Work out the finished part from the listing and answer in its coordinate system (mm). Give positions to 0.01 mm unless a question says otherwise; leave off trailing zeros. Loops run counter-clockwise (first coordinate to the right, second up) from the corner with the lowest first, then second, coordinate; pieces in that order, holes last. Notation, with made-up numbers: (34, 24.25) - (91, 24.25) arc R28 ccw to (91, 54.25) - close; hole circle Ø9 at (-15.75, 81). An arc over 180 degrees is marked (long way). One line per question, with ' | ' between items.
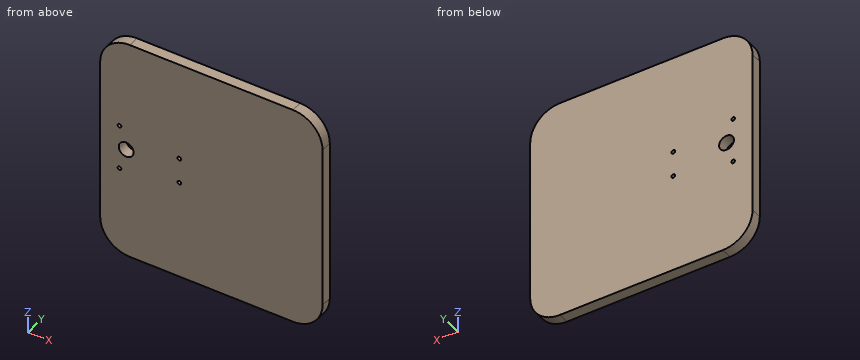
from build123d import *

# Parameters (mm, degrees)
SKETCH1_W               = 150
SKETCH1_H               = 150
BOSS_EXTRUDE1_DEPTH     = 7.5
CUT_EXTRUDE1_DEPTH      = 107.330851591
CUT_EXTRUDE1_DEPTH_BACK = 107.330851591
SKETCH2_R               = 1.25
SKETCH2_R_2             = 5
FILLET1_R               = 20


with BuildPart() as part:
    # Sketch1 → Boss-Extrude1 (new body)
    with BuildSketch(Plane(origin=(0, 0, 0), x_dir=(1, 0, 0), z_dir=(0, 1, 0))):
        Rectangle(SKETCH1_W, SKETCH1_H)
    extrude(amount=BOSS_EXTRUDE1_DEPTH)

    # Sketch2 → Cut-Extrude1 (cut, two sides: drawn at the far end of the back side and taken through both)
    with BuildSketch(Plane(origin=(0, 7.5, 0), x_dir=(1, 0, 0), z_dir=(0, 1, 0)).offset(-CUT_EXTRUDE1_DEPTH_BACK)):
        with Locations(Location((-61.985746634, -15.05, 0), (0, 0, 270))):
            Circle(SKETCH2_R)
        with Locations(Location((-61.985746634, 15.05, 0), (0, 0, 270))):
            Circle(SKETCH2_R)
        with Locations(Location((-21.585746634, 8.55, 0), (0, 0, 270))):
            Circle(SKETCH2_R)
        with Locations(Location((-21.585746634, -8.55, 0), (0, 0, 270))):
            Circle(SKETCH2_R)
        with Locations(Location((-57.485746634, 0, 0), (0, 0, 270))):
            Circle(SKETCH2_R_2)
    extrude(amount=CUT_EXTRUDE1_DEPTH + CUT_EXTRUDE1_DEPTH_BACK, mode=Mode.SUBTRACT)

    # Fillet1
    fillet1_edges = [part.edges().sort_by_distance(p)[0] for p in [
        (-75, 3.75, -75),
        (75, 3.75, -75),
        (75, 3.75, 75),
        (-75, 3.75, 75),
    ]]
    fillet(fillet1_edges, radius=FILLET1_R)


solid = part.part
1. Find section C-C on z = 65.5. Write down the section's boundary in (x, y), then the cut area to 3 significant figures.
Evaluation:
outline: (-72.02, 0) - (72.02, 0) - (72.02, 7.5) - (-72.02, 7.5) - close | area: 1,080 mm2
2. Consider L1, parallel to X at y = 3, z = -15.05; L2, parallel to X at y = 5.5, z = 0; L3, parallel to Z at x = -62, y = 7.25 (3 decimals). Determine where each line is inside the solid, lowest interval first.
Evaluation:
L1: -75 to -63.24, -60.74 to 75 | L2: -75 to -62.49, -52.49 to 75 | L3: -73.735 to -16.3, -13.8 to -2.15, 2.15 to 13.8, 16.3 to 73.735
3. Find section A-A on z = 0. Write down the section's boundary in (x, y).
Evaluation:
outline: (-75, 0) - (-62.49, 0) - (-62.49, 7.5) - (-75, 7.5) - close; (-52.49, 0) - (75, 0) - (75, 7.5) - (-52.49, 7.5) - close
4. A flat-ended cylindrical pin translates along its axis: pin 1 (11.5 mm diameter, centred on x = -57.49, z = 0, fed in from +Y). Find the tip coordinate at first contact, or state that the pin passes through.
Evaluation:
pin 1: y = 7.5
5. Find section B-B on y = 5. Write down the section's boundary in (x, z).
Evaluation:
outline: (-75, -55) arc R20 ccw to (-55, -75) - (55, -75) arc R20 ccw to (75, -55) - (75, 55) arc R20 ccw to (55, 75) - (-55, 75) arc R20 ccw to (-75, 55) - close; hole circle Ø2.5 at (-61.99, -15.05); hole circle Ø2.5 at (-61.99, 15.05); hole circle Ø10 at (-57.49, 0); hole circle Ø2.5 at (-21.59, -8.55); hole circle Ø2.5 at (-21.59, 8.55)
